Geometry: final body of the model. Coordinates: model frame, mm. A direction names the side the tool comes from. Round coordinates to 2 decimals unless told otherwise and drop trailing zeros. Write each loop counter-clockwise with the first axis right and the second up, starting at its lowest first coordinate (ties: lowest second). Pieces come first, ordered by that corner, then holes. Notation, with made-up numbers: (-13, 26) - (36, 26) arc R21 ccw to (36, 43) - close; hole circle Ø11 at (5, 40). An arc over 180 degrees is marked (long way). Write each question's results on one line, items separated by ' | '.
Autodesk Inventor part; units mm, degrees
ref_plane "YZ Plane" through (0, 0, 0) normal (1, 0, 0) x (0, 1, 0)
ref_plane "XZ Plane" through (0, 0, 0) normal (0, 1, 0) x (-1, 0, 0)
ref_plane "XY Plane" through (0, 0, 0) normal (0, 0, 1) x (1, 0, 0)
sketch "Szkic1" plane through (0, 0, 0) normal (0, 1, 0) x (-1, 0, 0)
  line L0 (0, 0) -> (100, 0)
  line L1 (100, 0) -> (100, -300)
  line L2 (100, -300) -> (0, -300)
  line L3 (0, -300) -> (0, 0)
  dimension "d0" = 300
  dimension "d1" = 100
sketch "Szkic2" plane through (0, 0, 0) normal (0, 1, 0) x (-1, 0, 0)
  line L0 (15, -15) -> (85, -15)
  line L1 (85, -15) -> (85, -285)
  line L2 (85, -285) -> (15, -285)
  line L3 (15, -285) -> (15, -15)
  point P0 (0, 0)
  dimension "d2" = 70
  dimension "d3" = 270
  dimension "d4" = 15
  dimension "d5" = 15
extrude "Wyciągnięcie proste1" add sketch "Szkic1" along normal blind 15
extrude "Wyciągnięcie proste2" cut sketch "Szkic2" along normal blind 15
fillet "Zaokrąglenie1" radius 2 8 edges at (-85, 7.5, -285) (-15, 7.5, -285) (-15, 7.5, -15) (-85, 7.5, -15) (-100, 7.5, 0) (-100, 7.5, -300) (0, 7.5, -300) (0, 7.5, 0)
sketch "Szkic3" plane through (0, 15, 0) normal (0, 1, 0) x (1, 0, 0)
  line L0 (0, 2) -> (0, 298)
  line L1 (-2, 300) -> (-98, 300)
  line L2 (-98, 0) -> (-2, 0)
  line L3 (-100, 298) -> (-100, 2)
  line L4 (-85, 17) -> (-85, 283)
  point P0 (0, 0)
  point P1 (-14, 295)
  point P2 (-14, 5)
  point P3 (-86, 295)
  point P4 (-86, 5)
  point P5 (-30, 100)
  point P6 (-100, 30)
  dimension "d12" = 5
  dimension "d13" = 5
  dimension "d14" = 5
  dimension "d18" = 5
  dimension "d32" = 14
  dimension "d33" = 14
  dimension "d34" = 14
  dimension "d35" = 14
hole "Otwór1" at (-14, 15, -295) at (-14, 15, -5) at (-86, 15, -295) at (-86, 15, -5) direction (0, -1, 0) diameter 5 depth 15
sketch "Szkic4" plane through (0, 15, 0) normal (0, 1, 0) x (1, 0, 0)
  line L0 (-100, 298) -> (-100, 2)
  line L1 (-100, 120) -> (100, 120)
  line L2 (100, 120) -> (100, 180)
  line L3 (100, 180) -> (-100, 180)
  line L4 (-100, 180) -> (-100, 120)
  line L5 (-98, 0) -> (-2, 0)
  point P0 (0, 0)
  point P1 (-100, 180)
  point P2 (-100, 30)
  dimension "d26" = 60
  dimension "d29" = 120
  dimension "d30" = 200
extrude "Wyciągnięcie proste3" add sketch "Szkic4" along normal blind 5
sketch "Szkic5" plane through (-100, 0, -298) normal (-1, 0, 0) x (0, 0, 1)
  line L0 (148, 20) -> (144.975, 20)
  line L1 (118, 20) -> (178, 20)
  line L2 (144.975, 20) -> (144.975, 22)
  line L3 (144.975, 22) -> (142.75, 22)
  line L4 (142.75, 22) -> (142.75, 25.5)
  line L5 (148, 26.5) -> (143.75, 26.5)
  line L6 (143.75, 26.5) -> (142.75, 25.5)
  line L7 (148, 20) -> (151.025, 20)
  line L8 (151.025, 20) -> (151.025, 22)
  line L9 (151.025, 22) -> (153.25, 22)
  line L10 (153.25, 22) -> (153.25, 25.5)
  line L11 (148, 26.5) -> (152.25, 26.5)
  line L12 (152.25, 26.5) -> (153.25, 25.5)
  line L13 (-2, 0) -> (-2, 15)
  point P0 (298, 0)
  point P1 (151.025, 20)
  dimension "d36" = 3.025
  dimension "d37" = 2
  dimension "d38" = 2.225
  dimension "d39" = 3.5
  dimension "d40" = 6.5
  dimension "d41" = 4.25
  dimension "d71" = 150
extrude "Wyciągnięcie proste4" add sketch "Szkic5" against normal blind 20
sketch "Szkic6" plane through (0, 20, 0) normal (0, 1, 0) x (1, 0, 0)
  line L0 (0, 2) -> (0, 120)
  line L1 (-100, 120) -> (100, 120)
  point P0 (0, 0)
  point P1 (5, 150)
  dimension "d51" = 5
  dimension "d69" = 30
hole "Otwór2" at (5, 20, -150) direction (0, -1, 0) diameter 3.424 end through all
sketch "Szkic7" plane through (0, 20, 0) normal (0, 1, 0) x (1, 0, 0)
  circle A0 centre (5, 150) radius 1.712
  line L0 (-100, 120) -> (100, 120)
  point P0 (0, 0)
  point P1 (62, 150)
  dimension "d52" = 57
  dimension "d70" = 30
hole "Otwór3" at (62, 20, -150) direction (0, -1, 0) diameter 7 end through all
sketch "Szkic8" plane through (0, 20, 0) normal (0, 1, 0) x (1, 0, 0)
  circle A0 centre (62, 150) radius 3.5
  line L0 (46.5, 134.5) -> (77.5, 165.5) construction
  line L1 (77.5, 134.5) -> (46.5, 165.5) construction
  point P0 (0, 0)
  dimension "d60" = 31
  dimension "d61" = 31
hole "Otwór4" at (46.5, 20, -165.5) at (77.5, 20, -165.5) at (77.5, 20, -134.5) at (46.5, 20, -134.5) direction (0, -1, 0) diameter 3.4 end through all
sketch "Szkic9" plane through (-98, 0, 0) normal (0, 0, 1) x (1, 0, 0)
  line L0 (33.475, 2) -> (39.475, 2)
  line L1 (39.475, 2) -> (39.475, 1.5)
  line L2 (39.475, 1.5) -> (33.475, 1.5)
  line L3 (33.475, 1.5) -> (33.475, 2)
  line L4 (98, 0) -> (98, 15)
  line L5 (0, 0) -> (96, 0)
  line L6 (-2, 15) -> (-2, 0)
  point P0 (33.475, 1.75)
  dimension "d72" = 6
  dimension "d73" = 0.5
  dimension "d75" = 1.5
  dimension "d78" = 35.475
extrude "Wyciągnięcie proste5" cut sketch "Szkic9" against normal through all
properties part number "podstawka_prowadzaca"
Q1. Pin query (flat end, axial travel): pin 1 (1.8 mm diameter, centred on x = -92, y = 23.5, fed in from -Z); pin 2 (2 mm diameter, centred on y = 24, z = -148.5, fed in from +X); pin 3 (4.5 mm diameter, centred on x = 5, z = -150, fed in from +Y). Return the tip coordinate at first contact, or that it passes through.
Answer block:
pin 1: z = -155.25 | pin 2: x = -80 | pin 3: y = 20
Q2. Ray query, line 1 along Z through (x, y) = (-86, 8); line 2 along X through (y, z) = (8.75, -295); line 3 along Z through (x, y) = (46.5, 16.45). Return the intervals inside material, ascending.
Answer block:
line 1: -300 to -297.5, -292.5 to -7.5, -2.5 to 0 | line 2: -100 to -88.5, -83.5 to -16.5, -11.5 to 0 | line 3: -180 to -167.2, -163.8 to -136.2, -132.8 to -120
Q3. Mould query, pull axis Y, two halves, no side actions, for faces 1 (the flat face through (-90, 26.5, -150)), 2 (the flat face through (-50, 7, -285)), 3 (the flat face through (-61, 1.5, -7)). Classes: pulls with the +Y half, pulls with the -Y half, needs draft (parallel to the pull), parting line crosses it, or undercut.
Answer block:
face 1: pulls with the +Y half | face 2: needs draft | face 3: undercut
Q4. Section query D-D, the plane x = -6. Return loops of the section in (y, z), plus the area to 3 significant figures.
Answer block:
outline: (0, -300) - (15, -300) - (15, -180) - (20, -180) - (20, -120) - (15, -120) - (15, 0) - (0, 0) - close | area: 4,800 mm2
Q5. Section query C-C, the plane y = 7. Return loops of the section in (x, z), plus the area to 3 significant figures.
Answer block:
outline: (-100, -298) arc R2 ccw to (-98, -300) - (-2, -300) arc R2 ccw to (0, -298) - (0, -2) arc R2 ccw to (-2, 0) - (-98, 0) arc R2 ccw to (-100, -2) - close; hole circle Ø5 at (-86, -295); hole circle Ø5 at (-86, -5); hole (-85, -283) arc R2 ccw to (-83, -285) - (-17, -285) arc R2 ccw to (-15, -283) - (-15, -17) arc R2 ccw to (-17, -15) - (-83, -15) arc R2 ccw to (-85, -17) - close; hole circle Ø5 at (-14, -295); hole circle Ø5 at (-14, -5) | area: 11,000 mm2
Q6. Section query A-A, the plane z = -112.5. Return loops of the section in (x, y), plus the area to 3 significant figures.
Answer block:
outline: (-100, 0) - (-85, 0) - (-85, 15) - (-100, 15) - close; (-15, 0) - (0, 0) - (0, 15) - (-15, 15) - close | area: 450 mm2
Q7. Access query for faces 4 (the flat face through (-13, 15, -249)), 5 (the flat face through (-61, 1.5, -292)), 6 (the flat face through (-50, 7, -15)), 7 (the flat face through (49, 15, -150)), 8 (the flat face through (-13, 15, -46)). Directions: +Z, -Z, +X, -X, +Y, -Y. A direction counts if a zero-diameter tool reaches every point of the face in a straight line with its end or side. Return the directions, or none.
Answer block:
face 4: -Z, +X, -X, +Y | face 5: +Z, -Z | face 6: +Y, -Y | face 7: +Z, -Z, +X, -Y | face 8: +Z, +X, -X, +Y
Q8. Section query B-B, the plane x = -37. Return loops of the section in (y, z), plus the area to 3 significant figures.
Answer block:
outline: (0, -300) - (15, -300) - (15, -285) - (0, -285) - close; (0, -15) - (15, -15) - (15, 0) - (0, 0) - close; (15, -180) - (20, -180) - (20, -120) - (15, -120) - close | area: 750 mm2
